from build123d import *

# Parameters (mm, degrees)
RESSALTO_EXTRUS_O2_DEPTH = 3
RESSALTO_EXTRUS_O3_START = 2
ESBO_O1_8_R              = 2
RESSALTO_EXTRUS_O3_DEPTH = 3
RESSALTO_EXTRUS_O4_DEPTH = 2


with BuildPart() as part:
    # Esbo_o1 → Ressalto-extrus_o2 (new body)
    with BuildSketch(Plane(origin=(0, 0, 0), x_dir=(1, 0, 0), z_dir=(0, 1, 0))):
        with BuildLine():
            ThreePointArc((-3, 0), (-2.121320344, -2.121320344), (0, -3))
            Line((0, -3), (41, -3))
            Line((41, -3), (52, -3))
            Line((52, -3), (93, -3))
            ThreePointArc((93, -3), (95.121320344, -2.121320344), (96, 0))
            Line((96, 0), (96, 38.5))
            Line((96, 38.5), (96, 49.5))
            Line((96, 49.5), (96, 88))
            ThreePointArc((96, 88), (95.121320344, 90.121320344), (93, 91))
            Line((93, 91), (52, 91))
            Line((52, 91), (41, 91))
            Line((41, 91), (0, 91))
            ThreePointArc((0, 91), (-2.121320344, 90.121320344), (-3, 88))
            Line((-3, 88), (-3, 0))
        make_face()
    extrude(amount=RESSALTO_EXTRUS_O2_DEPTH)

    # Esbo_o1_8 → Ressalto-extrus_o3 (add)
    # profile 1 of 2: a face of its own
    with BuildSketch(Plane(origin=(0, 0, 0), x_dir=(1, 0, 0), z_dir=(0, 1, 0)).offset(RESSALTO_EXTRUS_O3_START)):
        with BuildLine():
            Line((52, -3), (41, -3))
            Line((41, -3), (41, -13))
            ThreePointArc((41, -13), (41.585786438, -14.414213562), (43, -15))
            Line((43, -15), (50, -15))
            ThreePointArc((50, -15), (51.414213562, -14.414213562), (52, -13))
            Line((52, -13), (52, -3))
        make_face()
        with Locations(Location((46.5, -8.5, 0), (0, 0, 270))):
            Circle(ESBO_O1_8_R, mode=Mode.SUBTRACT)
    # profile 2 of 2: a face of its own
    with BuildSketch(Plane(origin=(0, 0, 0), x_dir=(1, 0, 0), z_dir=(0, 1, 0)).offset(RESSALTO_EXTRUS_O3_START)):
        with BuildLine():
            Line((41, 101), (41, 91))
            Line((41, 91), (52, 91))
            Line((52, 91), (52, 101))
            ThreePointArc((52, 101), (51.414213562, 102.414213562), (50, 103))
            Line((50, 103), (43, 103))
            ThreePointArc((43, 103), (41.585786438, 102.414213562), (41, 101))
        make_face()
        with Locations(Location((46.5, 96.5, 0), (0, 0, 270))):
            Circle(ESBO_O1_8_R, mode=Mode.SUBTRACT)
    extrude(amount=RESSALTO_EXTRUS_O3_DEPTH)

    # Esbo_o2 → Ressalto-extrus_o4 (add)
    with BuildSketch(Plane(origin=(0, 3, 0), x_dir=(1, 0, 0), z_dir=(0, 1, 0))):
        with BuildLine():
            Line((0, 90.960445131), (93, 90.960445131))
            ThreePointArc((93, 90.960445131), (95.121320344, 90.081765475), (96, 87.960445131))
            Line((96, 87.960445131), (96, 0))
            ThreePointArc((96, 0), (95.121320344, -2.121320344), (93, -3))
            Line((93, -3), (0, -3))
            ThreePointArc((0, -3), (-2.121320344, -2.121320344), (-3, 0))
            Line((-3, 0), (-3, 87.960445131))
            ThreePointArc((-3, 87.960445131), (-2.121320344, 90.081765475), (0, 90.960445131))
        make_face()
        with BuildLine():
            Line((1.5, 89.460445131), (91.5, 89.460445131))
            ThreePointArc((91.5, 89.460445131), (93.621320344, 88.581765475), (94.5, 86.460445131))
            Line((94.5, 86.460445131), (94.5, 1.5))
            ThreePointArc((94.5, 1.5), (93.621320344, -0.621320344), (91.5, -1.5))
            Line((91.5, -1.5), (1.5, -1.5))
            ThreePointArc((1.5, -1.5), (-0.621320344, -0.621320344), (-1.5, 1.5))
            Line((-1.5, 1.5), (-1.5, 86.460445131))
            ThreePointArc((-1.5, 86.460445131), (-0.621320344, 88.581765475), (1.5, 89.460445131))
        make_face(mode=Mode.SUBTRACT)
    extrude(amount=RESSALTO_EXTRUS_O4_DEPTH)


solid = part.part
Geometry: final body of the model. Coordinates: model frame, mm. A direction names the side the tool comes from. Round coordinates to 2 decimals unless told otherwise and drop trailing zeros. Order: outer loops, then holes, each group sorted by start corner. A loop starts at its lowest first (then second) coordinate and runs counter-clockwise, first axis right, second up.
Q1. Access query for faces 4 (the face through (-0.645, 3.986, -88.558)), 5 (the face through (47.6, 2, -98.4)), 6 (the face through (52, 3, -96)). Directions: +Z, -Z, +X, -X, +Y, -Y. A direction counts if a zero-diameter tool reaches every point of the face in a straight line with its end or side. Return the directions, or none.
Result sheet:
face 4: +Y
face 5: -Z, +X, -X, -Y
face 6: -Z, +X, +Y, -Y
Q2. Material intervals for probe 1 along X at (y, z) = (3.2, -75); probe 2 along X at (y, z) = (3.55, -96.5); probe 3 along Z at (x, y) = (82, 4.5), sorted ascending.
Result sheet:
probe 1: x = -3 to -1.5, 94.5 to 96
probe 2: x = 41 to 44.5, 48.5 to 52
probe 3: z = -90.96 to -89.46, 1.5 to 3
Q3. Mould query, pull axis X, two halves, no side actions, for faces 1 (the face through (52, 3, 8)), 2 (the face through (93.598, 3.986, -88.605)), 3 (the face through (46, 0, -45)). Classes: released by +X, released by -X, zero draft, split by the parting line, or undercut.
Result sheet:
face 1: released by +X
face 2: undercut
face 3: zero draft
Q4. Section A-A, the plane y = 4. Give the number of separate pieces and of enclosed holes in the cut face, and give its area (3 significant figures).
Result sheet:
separate pieces: 2
enclosed holes: 3
area: 805 mm2
Q5. Section B-B, the plane z = -96.5. Output: boundary loops of the cut face in (x, y), and give its area (3 significant figures).
Result sheet:
outline: (41, 2) - (44.5, 2) - (44.5, 5) - (41, 5) - close; (48.5, 2) - (52, 2) - (52, 5) - (48.5, 5) - close
area: 21.0 mm2
Q6. Pin query (flat end, axial travel): pin 1 (2 mm diameter, centred on x = 20.5, y = 2, fed in from +Z); pin 2 (0.9 mm diameter, centred on x = 43.5, y = 1.5, fed in from -Z); pin 3 (2.5 mm diameter, centred on y = 4, z = 6, fed in from +X); pin 4 (2 mm diameter, centred on x = 69, z = -43.5, fed in from -Y). Return the tip coordinate at first contact, or that it passes through.
Result sheet:
pin 1: stops at z = 3
pin 2: stops at z = -91
pin 3: stops at x = 52
pin 4: stops at y = 0
